Autodesk Inventor part; units mm, degrees
ref_plane "YZ Plane" through (0, 0, 0) normal (1, 0, 0) x (0, 1, 0)
ref_plane "XZ Plane" through (0, 0, 0) normal (0, 1, 0) x (-1, 0, 0)
ref_plane "XY Plane" through (0, 0, 0) normal (0, 0, 1) x (1, 0, 0)
sketch "Sketch1" plane through (0, 0, 0) normal (0, 1, 0) x (-1, 0, 0)
  circle A0 centre (0, 0) radius 12.5
  dimension "d0" = 25
extrude "Extrusion1" add sketch "Sketch1" along normal blind 33.5
hole "ReliefTop" at (0, 33.5, 0) direction (0, -1, 0) diameter 13.97 depth 0.254 countersink diameter 14.478 countersink angle 90
hole "ReliefBottom" at (0, 0, 0) direction (0, 1, 0) diameter 13.97 depth 0.254 countersink diameter 14.478 countersink angle 90
hole "MountBottomM6" at (0, 0.254, 0) direction (0, 1, 0) diameter 4.917 depth 7.366 tip angle 118 countersink diameter 5.508 countersink angle 90
hole "MountTopM4" at (0, 33.246, 0) direction (0, -1, 0) diameter 3.242 depth 14.478 tip angle 118 countersink diameter 3.808 countersink angle 90
sketch "Sketch2" plane through (0, 0, 0) normal (0, 0, 1) x (1, 0, 0)
  circle A0 centre (0, 20) radius 3
  line L0 (-12.5, 0) -> (12.5, 0)
  line L1 (0, -4.6) -> (0, 27.6)
  point P0 (0, 0)
  dimension "d49" = 6
  dimension "d50" = 20
extrude "Extrusion2" cut sketch "Sketch2" along normal through all both and the other way through all
chamfer "Chamfer1" distance 0.313 angle 45 2 edges at (-3, 19.9998, 12.1347) (-3, 19.9998, -12.1347)
extrude "Extrusion3" add sketch "Sketch2" along normal mid plane 14.84
equation "\"d1\" = height"
equation "\"d5\" = reliefMinor"
equation "\"d7\" = reliefMajor"
equation "\"d10\" = reliefDepth"
equation "\"d14\" = reliefMinor"
equation "\"d16\" = reliefMajor"
equation "\"d19\" = reliefDepth"
equation "\"d25\" = chamferM6"
equation "\"d28\" = depthM6"
equation "\"d40\" = chamferM4"
equation "\"d43\" = depthM4"
equation "\"reliefDepth\" = 0.254"
equation "\"reliefMinor\" = 13.97"
equation "\"reliefMajor\" = 14.478"
equation "\"chamferM6\" = 5.508"
equation "\"chamferM4\" = 3.808"
equation "\"depthM6\" = 7.366"
equation "\"depthM4\" = 14.478"
equation "\"height\" = 33.5"
properties part number "PLS-P642H0335A00_M" material "Stainless Steel"
Input: part model. Units: mm. Frame: model coordinates. A direction names the side the tool comes from. Give positions to 0.01 mm unless a question says otherwise; leave off trailing zeros. Order: outer loops, then holes, each group sorted by start corner. A loop starts at its lowest first (then second) coordinate and runs counter-clockwise, first axis right, second up. Notation, with made-up numbers: M 5,51.5 L 38,51.5 A19 ccw 38,71.5 Z; hole C 2,-2 d9. An arc over 180 degrees is marked long. One line per question, with ' | ' between items.
1) Draft query along X for faces 1 (the face through (-11.923, 16.516, -3.755)), 2 (the face through (-5.4, 0, -5.4)), 3 (the face through (0, 20, 7.42)), 4 (the face through (0.13, 8.84, -0.41)). Return one class per face: pulls with the +X half, pulls with the -X half, needs draft (parallel to the pull), parting line crosses it, or undercut.
Filled in:
face 1: parting line crosses it | face 2: needs draft | face 3: undercut | face 4: undercut
2) Section B-B on x = -10.75. Output: boundary loops of the cut face in (y, z), and give its area (3 significant figures).
Filled in:
outline: M 0,-6.38 L 33.5,-6.38 L 33.5,6.38 L 0,6.38 Z | area: 427 mm2
3) Section C-C on x = 9. Output: boundary loops of the cut face in (y, z), and give its area (3 significant figures).
Filled in:
outline: M 0,-8.67 L 33.5,-8.67 L 33.5,8.67 L 0,8.67 Z | area: 581 mm2
4) Access query for faces 5 (the face through (0, 23, 10)), 6 (the face through (0, 0.254, -3)), 7 (the face through (1.438, 27.671, 0.748)). Directions: +Z, -Z, +X, -X, +Y, -Y. A direction counts if a zero-diameter tool reaches every point of the face in a straight line with its end or side. Return the directions, or none.
Filled in:
face 5: +Z | face 6: -Y | face 7: +Y
5) Section A-A on y = 9.5. Output: boundary loops of the cut face in (x, z), and give its area (3 significant figures).
Filled in:
outline: C 0,0 d25 | area: 491 mm2
6) Contact query for flat-ended pins moving along their axis: P1, Ø6.5, axis at x = 0, z = 0, coming from the -Y side; P2, Ø1, axis at y = 18.5, z = 2, coming from the +X side; P3, Ø5, axis at x = 0, y = 20, coming from the -Z side. Output: stop coordinate, or through.
Filled in:
P1: stops at y = 0.25 | P2: stops at x = 12.41 | P3: stops at z = -7.42
7) Ray query, L1, parallel to Z at x = 0, y = 3; L2, parallel to Y at x = 0, z = 9.45; L3, parallel to Y at x = -4.5, z = -2.25. Return the intervals inside material, ascending.
Filled in:
L1: z = -12.5 to -2.46, 2.46 to 12.5 | L2: y = 0 to 17, 23 to 33.5 | L3: y = 0.25 to 33.25
